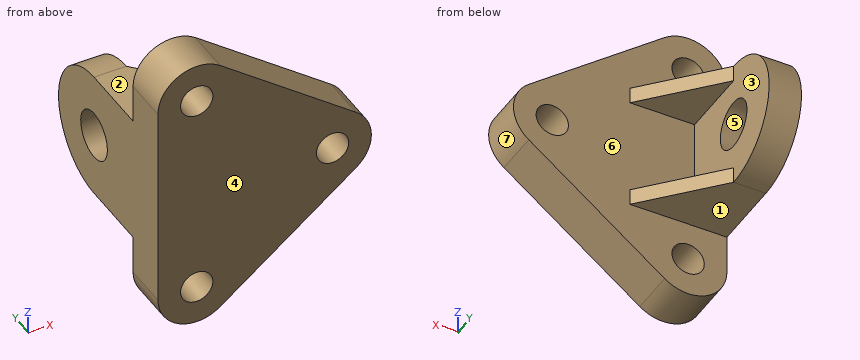
from build123d import *

# Parameters (mm, degrees)
SKETCH1_R           = 5
BOSS_EXTRUDE1_DEPTH = 14
SKETCH2_W           = 10
SKETCH2_H           = 40
BOSS_EXTRUDE2_DEPTH = 22
SKETCH4_R           = 20
BOSS_EXTRUDE3_DEPTH = 10
HOLE1_D             = 15
BOSS_EXTRUDE4_DEPTH = 5
BOSS_EXTRUDE5_DEPTH = 5


with BuildPart() as part:
    # Sketch1 → Boss-Extrude1 (new body)
    with BuildSketch(Plane(origin=(0, 0, 0), x_dir=(1, 0, 0), z_dir=(0, 1, 0))):
        with BuildLine():
            Line((-54, 32), (-54, -32))
            ThreePointArc((-54, -32), (-47.325869741, -42.753376749), (-34.727481417, -41.54518064))
            Line((-34.727481417, -41.54518064), (7.272518583, -9.54518064))
            ThreePointArc((7.272518583, -9.54518064), (12, 0), (7.272518583, 9.54518064))
            Line((7.272518583, 9.54518064), (-34.727481417, 41.54518064))
            ThreePointArc((-34.727481417, 41.54518064), (-47.325869741, 42.753376749), (-54, 32))
        make_face()
        with Locations(Location((-42, 32, 0), (0, 0, 270))):
            Circle(SKETCH1_R, mode=Mode.SUBTRACT)
        with Locations(Location((0, 0, 0), (0, 0, 270))):
            Circle(SKETCH1_R, mode=Mode.SUBTRACT)
        with Locations(Location((-42, -32, 0), (0, 0, 270))):
            Circle(SKETCH1_R, mode=Mode.SUBTRACT)
    extrude(amount=BOSS_EXTRUDE1_DEPTH)

    # Sketch2 → Boss-Extrude2 (add)
    with BuildSketch(Plane(origin=(0, 14, 0), x_dir=(1, 0, 0), z_dir=(0, 1, 0))):
        with Locations((-49, 0)):
            Rectangle(SKETCH2_W, SKETCH2_H)
    extrude(amount=BOSS_EXTRUDE2_DEPTH)

    # Sketch4 → Boss-Extrude3 (add)
    with BuildSketch(Plane.ZY.offset(54)):
        with Locations((0, 36)):
            Circle(SKETCH4_R)
    extrude(amount=-BOSS_EXTRUDE3_DEPTH)

    # Hole1 (through all)
    with Locations(Plane(origin=(-44, 0, 0), x_dir=(0, 0, -1), z_dir=(1, 0, 0))):
        with Locations((0, 36)):
            Hole(HOLE1_D / 2)

    # Sketch7 → Boss-Extrude4 (add)
    with BuildSketch(Plane.XY.offset(20)):
        Polygon((-44, 36), (-24, 14), (-44, 14), align=None)
    extrude(amount=-BOSS_EXTRUDE4_DEPTH)

    # Sketch8 → Boss-Extrude5 (add)
    with BuildSketch(Plane(origin=(0, 0, -20), x_dir=(-1, 0, 0), z_dir=(0, 0, -1))):
        Polygon((44, 36), (44, 14), (24, 14), align=None)
    extrude(amount=-BOSS_EXTRUDE5_DEPTH)


solid = part.part
Verification items for the finished model (mm, model axes). Face numbers are marked on the shaded views. A direction names the side the tool comes from. Give positions to 0.01 mm unless a question says otherwise; leave off trailing zeros. Loops run counter-clockwise (first coordinate to the right, second up) from the corner with the lowest first, then second, coordinate; pieces in that order, holes last. Notation, with made-up numbers: (34, 38) - (82, 38) arc R13 ccw to (82, 50) - close; hole circle Ø3 at (56, 74.25). An arc over 180 degrees is marked (long way). Write each question's results on one line, items separated by ' | '.
1) Sectioned sample at A-A on z = 0. Record the boundary of the cut face in (x, y), plus the area to 3 significant figures.
Solution:
outline: (-54, 0) - (-5, 0) - (-5, 14) - (-44, 14) - (-44, 28.5) - (-54, 28.5) - close; (-54, 43.5) - (-44, 43.5) - (-44, 56) - (-54, 56) - close; (5, 0) - (12, 0) - (12, 14) - (5, 14) - close | area: 1,050 mm2
2) Material ranges on L1, parallel to Y at x = -52, z = 0; L2, parallel to Y at x = -48, z = -37.5; L3, parallel to X at y = 7, z = -32, recorded low to high. Write a range as from..to.
Solution:
L1: 0..28.5, 43.5..56 | L2: 0..14 | L3: -54..-47, -37..-22.2
3) Depth check by flat-ended pin: P1, Ø17.5, axis at x = -35.5, y = 21.5, coming from the +Z side; P2, Ø8, axis at x = 0, z = 0, coming from the +Y side; P3, Ø10, axis at y = 50, z = 14, coming from the +X side; P4, Ø17.5, axis at x = -32.5, y = 25.5, coming from the -Z side. Enter the tip coordinate at first touch or a pass-through.
Solution:
P1: z = 43.83 | P2: through | P3: x = -44 | P4: z = -20
4) Sectioned sample at B-B on x = 0. Record the boundary of the cut face in (y, z).
Solution:
outline: (0, -15.09) - (14, -15.09) - (14, -5) - (0, -5) - close; (0, 5) - (14, 5) - (14, 15.09) - (0, 15.09) - close
5) Tool access check on the marked faces 1, 2, 3 and 4. Record the directions out of +Z, -Z, +X, -X, +Y, -Y that give a thin tool (end or side, any length) a straight path to the whole face; none if there is none.
Solution:
face 1: -Z, +X, -X, +Y | face 2: +Z, +X, -X, +Y | face 3: +X, +Y | face 4: +Z, -Z, +X, -X, -Y
6) Mould release check, pull along Y, two halves, no side actions. Record for the marked faces 5, 6 and 7: pulls with the +Y half, pulls with the -Y half, needs draft (parallel to the pull), parting line crosses it, or undercut.
Solution:
face 5: undercut | face 6: pulls with the +Y half | face 7: needs draft
7) Sectioned sample at D-D on x = -25. Record the boundary of the cut face in (y, z).
Solution:
outline: (0, -34.13) - (14, -34.13) - (14, -20) - (15.1, -20) - (15.1, -15) - (14, -15) - (14, 15) - (15.1, 15) - (15.1, 20) - (14, 20) - (14, 34.13) - (0, 34.13) - close
8) Sectioned sample at C-C on y = 7. Record the boundary of the cut face in (x, z).
Solution:
outline: (-54, -32) arc R12 ccw to (-34.73, -41.55) - (7.27, -9.55) arc R12 ccw to (7.27, 9.55) - (-34.73, 41.55) arc R12 ccw to (-54, 32) - close; hole circle Ø10 at (-42, -32); hole circle Ø10 at (-42, 32); hole circle Ø10 at (0, 0)
